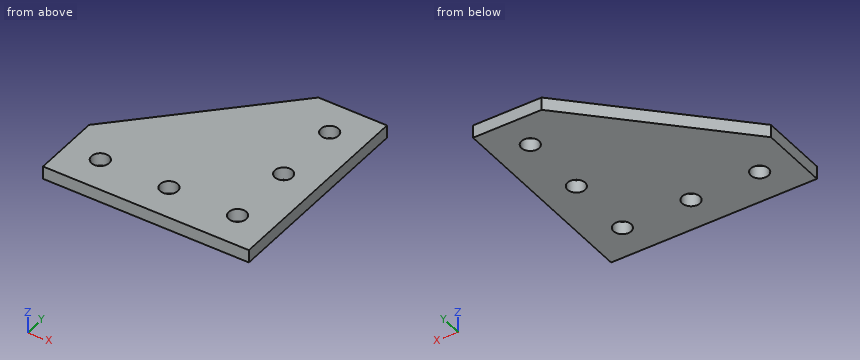
from build123d import *

# Parameters (mm, degrees)
EXTRUDE1_DEPTH  = 4.7625
SKETCH2_R       = 3.2639
SINGLE_90_DEPTH = 5.7625


with BuildPart() as part:
    # Sketch1 → Extrude1 (new body)
    with BuildSketch(Plane.XY):
        Polygon((25.4, 25.4), (50.8, 25.4), (50.8, -50.8), (-25.4, -50.8), (-25.4, -25.4), align=None)
    extrude(amount=-EXTRUDE1_DEPTH)

    # Sketch2 → single 90 (cut, through all)
    with BuildSketch(Plane(origin=(0, 0, -4.7625), x_dir=(-1, 0, 0), z_dir=(0, 0, -1))):
        with Locations((-38.1, -38.1)):
            Circle(SKETCH2_R)
        with Locations((-12.7, -38.1)):
            Circle(SKETCH2_R)
        with Locations((12.7, -38.1)):
            Circle(SKETCH2_R)
        with Locations((-38.1, -12.7)):
            Circle(SKETCH2_R)
        with Locations((-38.1, 12.7)):
            Circle(SKETCH2_R)
    extrude(amount=-SINGLE_90_DEPTH, mode=Mode.SUBTRACT)


solid = part.part
Geometry: final body of the model. Coordinates: model frame, mm. Give positions to 0.01 mm unless a question says otherwise; leave off trailing zeros. Order: outer loops, then holes, each group sorted by start corner. A loop starts at its lowest first (then second) coordinate and runs counter-clockwise, first axis right, second up. Notation, with made-up numbers: (38.25, 74.5) - (42.25, 74.5) arc R9 ccw to (42.25, 84.5) - close; hole circle Ø2 at (34.5, 45.25). An arc over 180 degrees is marked (long way). Use CSV: the item, a comma, the result in double quotes.
1. Section query A-A (x = -12.7). Output: boundary loops of the cut face in (y, z), plus the area to 3 significant figures.
Answers below:
outline,"(-50.8, -4.76) - (-41.36, -4.76) - (-41.36, 0) - (-50.8, 0) - close; (-34.84, -4.76) - (-12.7, -4.76) - (-12.7, 0) - (-34.84, 0) - close"
area,"150 mm2"
2. Section query D-D (y = 12.7). Output: boundary loops of the cut face in (x, z).
Answers below:
outline,"(12.7, -4.76) - (34.84, -4.76) - (34.84, 0) - (12.7, 0) - close; (41.36, -4.76) - (50.8, -4.76) - (50.8, 0) - (41.36, 0) - close"
3. Section query C-C (z = -3.5). Output: boundary loops of the cut face in (x, y).
Answers below:
outline,"(-25.4, -50.8) - (50.8, -50.8) - (50.8, 25.4) - (25.4, 25.4) - (-25.4, -25.4) - close; hole circle Ø6.53 at (-12.7, -38.1); hole circle Ø6.53 at (12.7, -38.1); hole circle Ø6.53 at (38.1, -38.1); hole circle Ø6.53 at (38.1, -12.7); hole circle Ø6.53 at (38.1, 12.7)"
4. Material intervals for line 1 along Y through (x, z) = (38.1, -1.6); line 2 along Y through (x, z) = (12.7, -1.75); line 3 along Y through (x, z) = (-15, -4.3), sorted ascending. Write a range as from..to.
Answers below:
line 1,"-50.8..-41.36, -34.84..-15.96, -9.44..9.44, 15.96..25.4"
line 2,"-50.8..-41.36, -34.84..12.7"
line 3,"-50.8..-40.42, -35.78..-15"
5. Section query B-B (y = -38.1). Output: boundary loops of the cut face in (x, z).
Answers below:
outline,"(-25.4, -4.76) - (-15.96, -4.76) - (-15.96, 0) - (-25.4, 0) - close; (-9.44, -4.76) - (9.44, -4.76) - (9.44, 0) - (-9.44, 0) - close; (15.96, -4.76) - (34.84, -4.76) - (34.84, 0) - (15.96, 0) - close; (41.36, -4.76) - (50.8, -4.76) - (50.8, 0) - (41.36, 0) - close"
6. Contact query for flat-ended pins moving along their axis: pin 1 (12 mm diameter, centred on x = 0.5, y = 2.5, fed in from -Z); pin 2 (6 mm diameter, centred on x = 38.1, y = -38.1, fed in from +Z). Output: stop coordinate, or through.
Answers below:
pin 1,"z = -4.76"
pin 2,"through"
